The listing builds one solid part. Answer for the finished solid, in the listing's coordinates (mm). Face numbers are marked on the shaded views. A direction names the side the tool comes from. Give positions to 0.01 mm unless a question says otherwise; leave off trailing zeros. Write each loop counter-clockwise with the first axis right and the second up, starting at its lowest first coordinate (ties: lowest second). Pieces come first, ordered by that corner, then holes. Notation, with made-up numbers: (89.5, 16.25) - (112.5, 16.25) arc R10 ccw to (112.5, 34.25) - close; hole circle Ø9 at (1, 87). An arc over 180 degrees is marked (long way). Return JSON: item names as keys, results as strings.
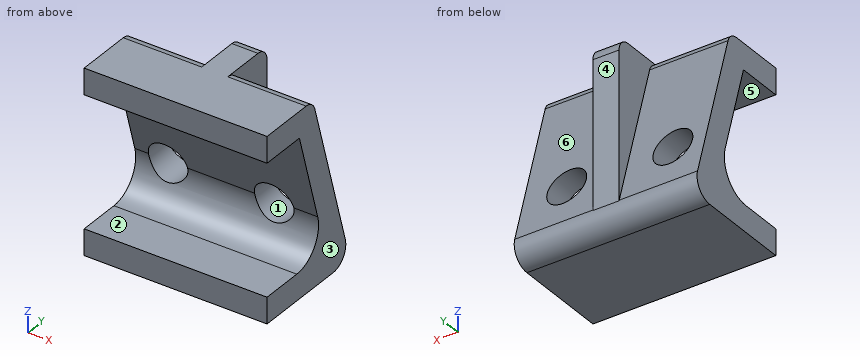
from build123d import *

# Parameters (mm, degrees)
BOSS_EXTRUDE1_DEPTH = 35
BOSS_EXTRUDE2_REACH = 91.5
SKETCH4_W           = 9.999142244
SKETCH4_H           = 17.913024492
CUT_EXTRUDE1_REACH  = 91.5
SKETCH6_R           = 7.5
FILLET2_R           = 5


with BuildPart() as part:
    # Sketch2 → Boss-Extrude1 (new, symmetric)
    with BuildSketch(Plane(origin=(0, 0, 0), x_dir=(0, 0, -1), z_dir=(1, 0, 0))):
        with BuildLine():
            Line((0, 25.295092448), (0, 0))
            Line((0, 0), (10, 0))
            Line((10, 0), (10, 17.831828992))
            Line((10, 17.831828992), (44.647504272, 27.912868223))
            ThreePointArc((44.647504272, 27.912868223), (55.203126101, 25.988336757), (60, 16.390682129))
            Line((60, 16.390682129), (60, 0))
            Line((60, 0), (70, 0))
            Line((70, 0), (70, 36.418950493))
            ThreePointArc((70, 36.418950493), (67.19828686, 42.020234938), (61.035889303, 43.137750175))
            Line((61.035889303, 43.137750175), (0, 25.295092448))
        make_face()
    extrude(amount=BOSS_EXTRUDE1_DEPTH, both=True)

    # Sketch4 → Boss-Extrude2 (add, up to next)
    with BuildSketch(Plane.XY, mode=Mode.PRIVATE) as boss_extrude2_sk1:
        with Locations((0, 34.251604694)):
            Rectangle(SKETCH4_W, SKETCH4_H)
    boss_extrude2_tool1 = extrude(boss_extrude2_sk1.sketch, amount=-BOSS_EXTRUDE2_REACH, mode=Mode.PRIVATE) - part.part
    add(boss_extrude2_tool1.solids().sort_by_distance((0, 34.251605, 0))[0])

    # Cut-Extrude1: up to this plane
    cut_extrude1_end = Plane(origin=(35, 43.137750175, -61.035889303), z_dir=(0, -0.9598285260414122, -0.280587242399169))
    # Sketch6 → Cut-Extrude1 (cut, up to the surface)
    with BuildSketch(Plane(origin=(0, 0, 0), x_dir=(1, 0, 0), z_dir=(0, 1, 0)), mode=Mode.PRIVATE) as cut_extrude1_sk1:
        with Locations(Location((18.359997259, 44.938878516, 0), (0, 0, 182.226493381))):
            Circle(SKETCH6_R)
    cut_extrude1_tool1 = split(extrude(cut_extrude1_sk1.sketch, amount=CUT_EXTRUDE1_REACH, mode=Mode.PRIVATE), bisect_by=cut_extrude1_end, keep=Keep.BOTH, mode=Mode.PRIVATE)
    add(cut_extrude1_tool1.solids().sort_by_distance((18.359997, 0, -44.938879))[0], mode=Mode.SUBTRACT)
    # Sketch6 → Cut-Extrude1 (cut, up to the surface)
    with BuildSketch(Plane(origin=(0, 0, 0), x_dir=(1, 0, 0), z_dir=(0, 1, 0)), mode=Mode.PRIVATE) as cut_extrude1_sk2:
        with Locations(Location((-22.276796675, 44.938878516, 0), (0, 0, 182.226493381))):
            Circle(SKETCH6_R)
    cut_extrude1_tool2 = split(extrude(cut_extrude1_sk2.sketch, amount=CUT_EXTRUDE1_REACH, mode=Mode.PRIVATE), bisect_by=cut_extrude1_end, keep=Keep.BOTH, mode=Mode.PRIVATE)
    add(cut_extrude1_tool2.solids().sort_by_distance((-22.276797, 0, -44.938879))[0], mode=Mode.SUBTRACT)

    # Fillet2
    fillet2_edges = [part.edges().sort_by_distance(p)[0] for p in [
        (19.999785561, 25.295092448, 0),
        (-19.999785561, 25.295092448, 0),
        (0, 43.20811694, 0),
    ]]
    fillet(fillet2_edges, radius=FILLET2_R)


solid = part.part
Item 1: A cutting plane is placed at B-B on z = -51.5. Determine the outline of the cut face in (x, y).
Answer below:
{"outline": "(-35, 27.87) - (-25.91, 27.87) - (-25.91, 40.35) - (-35, 40.35) - close; (-18.64, 27.87) - (14.73, 27.87) - (14.73, 40.35) - (5, 40.35) - (5, 43.21) - (-5, 43.21) - (-5, 40.35) - (-18.64, 40.35) - close; (21.99, 27.87) - (35, 27.87) - (35, 40.35) - (21.99, 40.35) - close"}
Item 2: A cutting plane is placed at A-A on y = 7. Determine the outline of the cut face in (x, z), then the cut area to 3 significant figures.
Answer below:
{"outline": "(-35, -70) - (35, -70) - (35, -60) - (-35, -60) - close; (-35, -10) - (35, -10) - (35, 0) - (-35, 0) - close", "area": "1,400 mm²"}
Item 3: For the marked faces 4, 5 and 6, determine the directions among +Z, -Z, +X, -X, +Y, -Y from which every point of the face is accessible in a straight line to the end or side of a thin tool.
Answer below:
{"face 4": "+Z, +X, -X, +Y", "face 5": "+X, -X, -Y", "face 6": "+Z, +X, +Y"}
Item 4: Consider L1, parallel to Z at x = 29.5, y = 14; L2, parallel to Z at x = 14, y = 17.5; L3, parallel to X at y = 36, z = -29. Determine where each line is inside the solid, lowest interval first.
Answer below:
{"L1": "z = -70 to -60, -10 to 0", "L2": "z = -70 to -59.95, -10 to 0", "L3": "x = -5 to 5"}
Item 5: The mould has two halves that part along X. Classify the marked faces 1, 2 and 3: +X half, -X half, draft (parallel to the pull), parting line (faces both ways), or undercut.
Answer below:
{"face 1": "undercut", "face 2": "draft", "face 3": "+X half"}
Item 6: A cutting plane is placed at C-C on x = 30. Determine the outline of the cut face in (y, z).
Answer below:
{"outline": "(0, -70) - (36.42, -70) arc R7 ccw to (43.14, -61.04) - (26.35, -3.6) arc R5 ccw to (21.55, 0) - (0, 0) - (0, -10) - (17.83, -10) - (27.91, -44.65) arc R12 cw to (16.39, -60) - (0, -60) - close"}
Item 7: A cutting plane is placed at D-D on x = -28. Determine the outline of the cut face in (y, z), then the cut area to 3 significant figures.
Answer below:
{"outline": "(0, -70) - (36.42, -70) arc R7 ccw to (43.14, -61.04) - (39.85, -49.79) - (28.26, -49.79) arc R12 cw to (16.39, -60) - (0, -60) - close; (0, -10) - (17.83, -10) - (26.59, -40.09) - (37.02, -40.09) - (26.35, -3.6) arc R5 ccw to (21.55, 0) - (0, 0) - close", "area": "1,160 mm²"}
Item 8: Flat-ended cylindrical pins translate along their axes: P1, Ø5, axis at x = 2, z = -19.5, coming from the +Y side; P2, Ø12, axis at x = 18.36, z = -44.94, coming from the +Y side. Find the tip coordinate at first contact, or state that the pin passes through.
Answer below:
{"P1": "stops at y = 43.21", "P2": "passes through"}
